Check sheet for the modelled part. Datum: model origin and axes. Units: mm. A direction names the side the tool comes from. Round coordinates to 2 decimals unless told otherwise and drop trailing zeros. Write each loop counter-clockwise with the first axis right and the second up, starting at its lowest first coordinate (ties: lowest second). Pieces come first, ordered by that corner, then holes. Notation, with made-up numbers: (42.5, 70.5) - (64.5, 70.5) arc R30 ccw to (64.5, 108.5) - close; hole circle Ø6 at (46.5, 76). An arc over 180 degrees is marked (long way). Answer as a JSON object with one key per item and string values. Group by question number.
Item 1: Sectioned sample at B-B on z = 0. Record the boundary of the cut face in (x, y), plus the area to 3 significant figures.
Item 2: Sectioned sample at A-A on y = -109. Record the boundary of the cut face in (x, z), plus the area to 3 significant figures.
Item 3: Sectioned sample at C-C on y = 0. Record the boundary of the cut face in (x, z), plus the area to 3 significant figures.
Item 4: Sectioned sample at D-D on x = 4. Record the boundary of the cut face in (y, z), plus the area to 3 significant figures.
Item 5: Release check for a two-part mould opening along Z. For faces 1 (the cylindrical face through (10.507, -3.517, -79.923)), 2 (the cylindrical face through (22.97, -5.5, -124.88)), 3 (the flat face through (25, 92, 28)) record: pulls with the +Z half, pulls with the -Z half, needs draft (parallel to the pull), parting line crosses it, or undercut.
Item 6: Thickness scan on line 1 (Y direction, x = 10.3, z = 0); line 2 (X direction, y = -65.5, z = 87); line 3 (X direction, y = 10, z = 62). Record the ranges inside material, lowest first.
Item 7: Set-up check for faces 4 (the cylindrical face through (22.972, 114.453, -0.716)), 5 (the flat face through (21, 92, -28)), 6 (the flat face through (0, -1, 1)): record each of +Z, -Z, +X, -X, +Y, -Y from which the full face is reachable in a straight line by a thin tool's end or side.
Item 8: Gauge pin test, flat ends, axial feed: P1, Ø1, axis at x = 11, y = 41, coming from the +Z side; P2, Ø1, axis at y = -50.5, z = -59, coming from the -X side; P3, Ø1, axis at x = 4, y = -9, coming from the +Z side; P4, Ø10, axis at y = -54.5, z = -94.4, coming from the +X side. Record the tip position at first contact, or that the pin passes through.
```python
from build123d import *

# Parameters (mm, degrees)
SKETCH2_R          = 5.5
CUT_EXTRUDE1_DEPTH = 179.535710728
CIRPATTERN1_COUNT  = 6


with BuildPart() as part:
    # Sketch1 → Revolve1 (revolve)
    with BuildSketch(Plane.XY, mode=Mode.PRIVATE) as revolve1_sk:
        with BuildLine():
            Line((0, 0), (0, 70))
            ThreePointArc((0, 70), (2.928932188, 77.071067812), (10, 80))
            Line((10, 80), (11, 80))
            ThreePointArc((11, 80), (20.899494937, 84.100505063), (25, 94))
            Line((25, 94), (25, 125))
            Line((25, 125), (21, 125))
            Line((21, 125), (21, 94))
            ThreePointArc((21, 94), (18.071067812, 86.928932188), (11, 84))
            Line((11, 84), (10, 84))
            ThreePointArc((10, 84), (0.100505063, 79.899494937), (-4, 70))
            Line((-4, 70), (-4, 0))
            Line((-4, 0), (0, 0))
        make_face()
    revolve(revolve1_sk.sketch.rotate(Axis((-4, 0, 0), (1, 0, 0)), 90), axis=Axis((-4, 0, 0), (1, 0, 0)))

    # Sketch2 → Cut-Extrude1 (cut, through all)
    with BuildSketch(Plane.ZY.offset(-21)):
        with Locations((0, 109)):
            Circle(SKETCH2_R)
    cut_extrude1 = extrude(amount=-CUT_EXTRUDE1_DEPTH, mode=Mode.SUBTRACT)

    # CirPattern1: Cut-Extrude1 ×6 about axis
    cirpattern1_axis = Axis((0, 0, 0), (1, 0, 0))
    for i in range(1, CIRPATTERN1_COUNT):
        add(cut_extrude1.rotate(cirpattern1_axis, i * 360 / CIRPATTERN1_COUNT), mode=Mode.SUBTRACT)


solid = part.part
```
Completed:
{
 "1": {"outline": "(-4, -70) arc R14 ccw to (10, -84) - (11, -84) arc R10 cw to (21, -94) - (21, -103.5) - (25, -103.5) - (25, -94) arc R14 ccw to (11, -80) - (10, -80) arc R10 cw to (0, -70) - (0, 70) arc R10 cw to (10, 80) - (11, 80) arc R14 ccw to (25, 94) - (25, 103.5) - (21, 103.5) - (21, 94) arc R10 cw to (11, 84) - (10, 84) arc R14 ccw to (-4, 70) - close; (21, -125) - (25, -125) - (25, -114.5) - (21, -114.5) - close; (21, 114.5) - (25, 114.5) - (25, 125) - (21, 125) - close", "area": "1,030 mm²"},
 "2": {"outline": "(21, -61.19) - (25, -61.19) - (25, -5.5) - (21, -5.5) - close; (21, 5.5) - (25, 5.5) - (25, 61.19) - (21, 61.19) - close", "area": "446 mm²"},
 "3": {"outline": "(-4, -70) arc R14 ccw to (10, -84) - (11, -84) arc R10 cw to (21, -94) - (21, -125) - (25, -125) - (25, -94) arc R14 ccw to (11, -80) - (10, -80) arc R10 cw to (0, -70) - (0, 70) arc R10 cw to (10, 80) - (11, 80) arc R14 ccw to (25, 94) - (25, 125) - (21, 125) - (21, 94) arc R10 cw to (11, 84) - (10, 84) arc R14 ccw to (-4, 70) - close", "area": "1,120 mm²"},
 "4": {"outline": "circle Ø165.3 at (0, 0); hole circle Ø156 at (0, 0)", "area": "2,350 mm²"},
 "5": {"face 1": "undercut", "face 2": "parting line crosses it", "face 3": "needs draft"},
 "6": {"line 1": "-84 to -80, 80 to 84", "line 2": "21 to 25", "line 3": "-4 to 0"},
 "7": {"face 4": "+X, -X", "face 5": "-X", "face 6": "+X"},
 "8": {"P1": "z = 73.59", "P2": "x = -2.03", "P3": "z = 82.39", "P4": "through"}
}
